```python
from build123d import *

# Parameters (mm, degrees)
SKETCH1_W                    = 76.2
SKETCH1_H                    = 25.4
BOSS_EXTRUDE1_DEPTH          = 1.5875
F_12_0MM_DOWEL_HOLE1_D       = 12
SKETCH5_W                    = 4.7625
SKETCH5_H                    = 25.4
BOSS_EXTRUDE2_DEPTH          = 3.175
M2_5X0_45_TAPPED_HOLE1_D     = 2.05
M2_5X0_45_TAPPED_HOLE1_DEPTH = 3.999992
M2_5X0_45_TAPPED_HOLE1_TIP   = 0.615882135
M2_5X0_45_TAPPED_HOLE2_D     = 2.05
M2_5X0_45_TAPPED_HOLE2_DEPTH = 3.999992
M2_5X0_45_TAPPED_HOLE2_TIP   = 0.615882135
CUT_EXTRUDE1_DEPTH           = 41.286233691
FILLET1_R                    = 1.5875


with BuildPart() as part:
    # Sketch1 → Boss-Extrude1 (new, symmetric)
    with BuildSketch(Plane(origin=(0, 0, 0), x_dir=(1, 0, 0), z_dir=(0, 1, 0))):
        Rectangle(SKETCH1_W, SKETCH1_H)
    extrude(amount=BOSS_EXTRUDE1_DEPTH, both=True)

    # Ø12.0mm Dowel Hole1 (through all)
    with Locations(Plane(origin=(0, 1.5875, 0), x_dir=(1, 0, 0), z_dir=(0, 1, 0))):
        with Locations((0, 0)):
            Hole(F_12_0MM_DOWEL_HOLE1_D / 2)

    # Sketch5 → Boss-Extrude2 (add)
    with BuildSketch(Plane(origin=(0, 1.5875, 0), x_dir=(1, 0, 0), z_dir=(0, 1, 0))):
        with Locations((-35.71875, 0)):
            Rectangle(SKETCH5_W, SKETCH5_H)
    boss_extrude2 = extrude(amount=BOSS_EXTRUDE2_DEPTH)

    # Mirror1: Boss-Extrude2 across plane
    add(boss_extrude2.mirror(Plane(origin=(0, 0, 0), x_dir=(0, 0, 1), z_dir=(1, 0, 0))))

    # M2.5x0.45 Tapped Hole1
    with Locations(Plane.ZY.offset(38.1)):
        with Locations((7.9375, 1.5875), (-7.9375, 1.5875)):
            Hole(M2_5X0_45_TAPPED_HOLE1_D / 2, depth=M2_5X0_45_TAPPED_HOLE1_DEPTH)
            with Locations((0, 0, -(M2_5X0_45_TAPPED_HOLE1_DEPTH + M2_5X0_45_TAPPED_HOLE1_TIP / 2))):  # 118° drill point
                Cone(0, M2_5X0_45_TAPPED_HOLE1_D / 2, M2_5X0_45_TAPPED_HOLE1_TIP, mode=Mode.SUBTRACT)

    # M2.5x0.45 Tapped Hole2
    with Locations(Plane(origin=(38.1, 0, 0), x_dir=(0, 0, -1), z_dir=(1, 0, 0))):
        with Locations((-7.9375, 1.5875), (7.9375, 1.5875)):
            Hole(M2_5X0_45_TAPPED_HOLE2_D / 2, depth=M2_5X0_45_TAPPED_HOLE2_DEPTH)
            with Locations((0, 0, -(M2_5X0_45_TAPPED_HOLE2_DEPTH + M2_5X0_45_TAPPED_HOLE2_TIP / 2))):  # 118° drill point
                Cone(0, M2_5X0_45_TAPPED_HOLE2_D / 2, M2_5X0_45_TAPPED_HOLE2_TIP, mode=Mode.SUBTRACT)

    # Sketch12 → Cut-Extrude1 (cut, through all)
    with BuildSketch(Plane(origin=(0, 1.5875, 0), x_dir=(1, 0, 0), z_dir=(0, 1, 0))):
        with BuildLine():
            Line((-30.95625, 7.9375), (-30.95625, -7.9375))
            Line((-30.95625, -7.9375), (-9.461426623, -7.9375))
            ThreePointArc((-9.461426623, -7.9375), (-12.35, 0), (-9.461426623, 7.9375))
            Line((-9.461426623, 7.9375), (-30.95625, 7.9375))
        make_face()
    cut_extrude1 = extrude(amount=-CUT_EXTRUDE1_DEPTH, mode=Mode.SUBTRACT)

    # Mirror2: Cut-Extrude1 across plane
    add(cut_extrude1.mirror(Plane(origin=(0, 0, 0), x_dir=(0, 0, 1), z_dir=(1, 0, 0))), mode=Mode.SUBTRACT)

    # Fillet1
    fillet1_edges = [part.edges().sort_by_distance(p)[0] for p in [
        (-30.95625, 0, -7.9375),
        (-9.461426623, 0, -7.9375),
        (-9.461426623, 0, 7.9375),
        (-30.95625, 0, 7.9375),
        (9.461426623, 0, -7.9375),
        (30.95625, 0, -7.9375),
        (30.95625, 0, 7.9375),
        (9.461426623, 0, 7.9375),
    ]]
    fillet(fillet1_edges, radius=FILLET1_R)


solid = part.part
```
Geometry check sheet. Reference: the model listing, model coordinates, mm. A direction names the side the tool comes from. Coordinates: 2 decimals unless noted, no trailing zeros. Write each loop counter-clockwise with the first axis right and the second up, starting at its lowest first coordinate (ties: lowest second). Pieces come first, ordered by that corner, then holes. Notation, with made-up numbers: M 83.5,82 L 109.5,82 A13 cw 109.5,92 Z; hole C -14.5,66 d8. An arc over 180 degrees is marked long. Answer as a JSON object with one key per item and string values.
1. Section check A-A, the plane z = 0. Enter the section's corners in (x, y).
Answers below:
{"outline": "M -38.1,-1.59 L -30.96,-1.59 L -30.96,1.59 L -33.34,1.59 L -33.34,4.76 L -38.1,4.76 Z; M -12.35,-1.59 L -6,-1.59 L -6,1.59 L -12.35,1.59 Z; M 6,-1.59 L 12.35,-1.59 L 12.35,1.59 L 6,1.59 Z; M 30.96,-1.59 L 38.1,-1.59 L 38.1,4.76 L 33.34,4.76 L 33.34,1.59 L 30.96,1.59 Z"}
2. Scan lines: L1, parallel to X at y = 2.75, z = -5; L2, parallel to Z at x = 0, y = -0.25; L3, parallel to Z at x = 16, y = 0. Record each from-to range of solid material in increasing order.
Answers below:
{"L1": "x = -38.1 to -33.34, 33.34 to 38.1", "L2": "z = -12.7 to -6, 6 to 12.7", "L3": "z = -12.7 to -7.94, 7.94 to 12.7"}
3. Section check B-B, the plane x = 27.5. Enter the section's corners in (y, z).
Answers below:
{"outline": "M -1.59,-12.7 L 1.59,-12.7 L 1.59,-7.94 L -1.59,-7.94 Z; M -1.59,7.94 L 1.59,7.94 L 1.59,12.7 L -1.59,12.7 Z"}
4. Section check D-D, the plane z = 10.25. Enter the section's corners in (x, y), plus the area to 3 significant figures.
Answers below:
{"outline": "M -38.1,-1.59 L 38.1,-1.59 L 38.1,4.76 L 33.34,4.76 L 33.34,1.59 L -33.34,1.59 L -33.34,4.76 L -38.1,4.76 Z", "area": "272 mm²"}
5. Draft check along Y on faces 1 (the flat face through (-30.956, 0, 0)), 2 (the cylindrical face through (36.07, 1.63, -8.96)), 3 (the flat face through (-36, 4.762, 0)). Enter one of: released by +Y, released by -Y, zero draft, split by the parting line, or undercut.
Answers below:
{"face 1": "zero draft", "face 2": "undercut", "face 3": "released by +Y"}
6. Go/stop test with flat-tipped pins: pin 1 Ø1.2 at (y, z) = (1.59, -7.94) entering from +X; pin 2 Ø8 at (x, z) = (17.5, -7) entering from +Y; pin 3 Ø1.6 at (y, z) = (1.59, 7.94) entering from +X. Record where each tip stops, or that it passes through.
Answers below:
{"pin 1": "stops at x = 33.85", "pin 2": "stops at y = 1.59", "pin 3": "stops at x = 33.97"}
7. Tool access check on faces 4 (the flat face through (7, 1.588, 0)), 5 (the cylindrical face through (36, 2, 7)), 6 (the cylindrical face through (12.35, 0.02, 0.08)). Record the directions out of +Z, -Z, +X, -X, +Y, -Y that give a thin tool (end or side, any length) a straight path to the whole face; none if there is none.
Answers below:
{"face 4": "+Z, -Z, +Y", "face 5": "+X", "face 6": "+Y, -Y"}
8. Section check C-C, the plane y = 4. Enter the section's corners in (x, z), plus the area to 3 significant figures.
Answers below:
{"outline": "M -38.1,-12.7 L -33.34,-12.7 L -33.34,12.7 L -38.1,12.7 Z; M 33.34,-12.7 L 38.1,-12.7 L 38.1,12.7 L 33.34,12.7 Z", "area": "242 mm²"}
